Geometry: see drawing. Coordinates: mm, zero at the bounding-box minimum. A direction names the side the tool comes from. Coordinates: 2 decimals unless noted, no trailing zeros. Write each loop counter-clockwise with the first axis right and the second up, starting at its lowest first coordinate (ties: lowest second). Pieces come first, ordered by that corner, then holes. Notation, with made-up numbers: M -29.5,22.25 L -10.5,22.25 A24 ccw -10.5,59.25 Z; hole C 19,19.5 d3. An arc over 180 degrees is marked long. One line per item, written item: value. Start each with the question number.
Item 1: Mould query, pull axis Y, two halves, no side actions, for the marked faces 1, 2 and 3. Classes: released by +Y, released by -Y, zero draft, split by the parting line, or undercut.
Item 2: Cut plane C-C, the plane y = 10. Output: boundary loops of the cut face in (x, z), then the cut area to 3 significant figures.
Item 3: Cut plane D-D, the plane x = 5. Output: boundary loops of the cut face in (y, z), then the cut area to 3 significant figures.
Item 4: Set-up query: the marked faces 4, 5, 6 and 7. Return all of +Z, -Z, +X, -X, +Y, -Y with unobstructed straight access to the full face (end or side cutting, diameter ignored); none if empty.
Item 5: Cut plane A-A, the plane x = 8.75. Output: boundary loops of the cut face in (y, z).
Item 6: Pin query (flat end, axial travel): P1, Ø3.5, axis at y = 9.5, z = 4, coming from the -X side; P2, Ø3, axis at x = 7, y = 6.5, coming from the +Z side; P3, Ø6.5, axis at x = 9.5, y = 9.5, coming from the +Z side; P4, Ø4, axis at x = 15, z = 12.5, coming from the -Y side. Return the tip coordinate at first contact, or that it passes through.
Item 7: Ray query, L1, parallel to X at y = 7.25, z = 18.5; L2, parallel to X at y = 1.5, z = 20.7; L3, parallel to Y at x = 3.25, z = 4. Return the intervals inside material, ascending. Write a range as from..to.
Item 8: Cut plane B-B, the plane z = 21.25. Output: boundary loops of the cut face in (x, y).
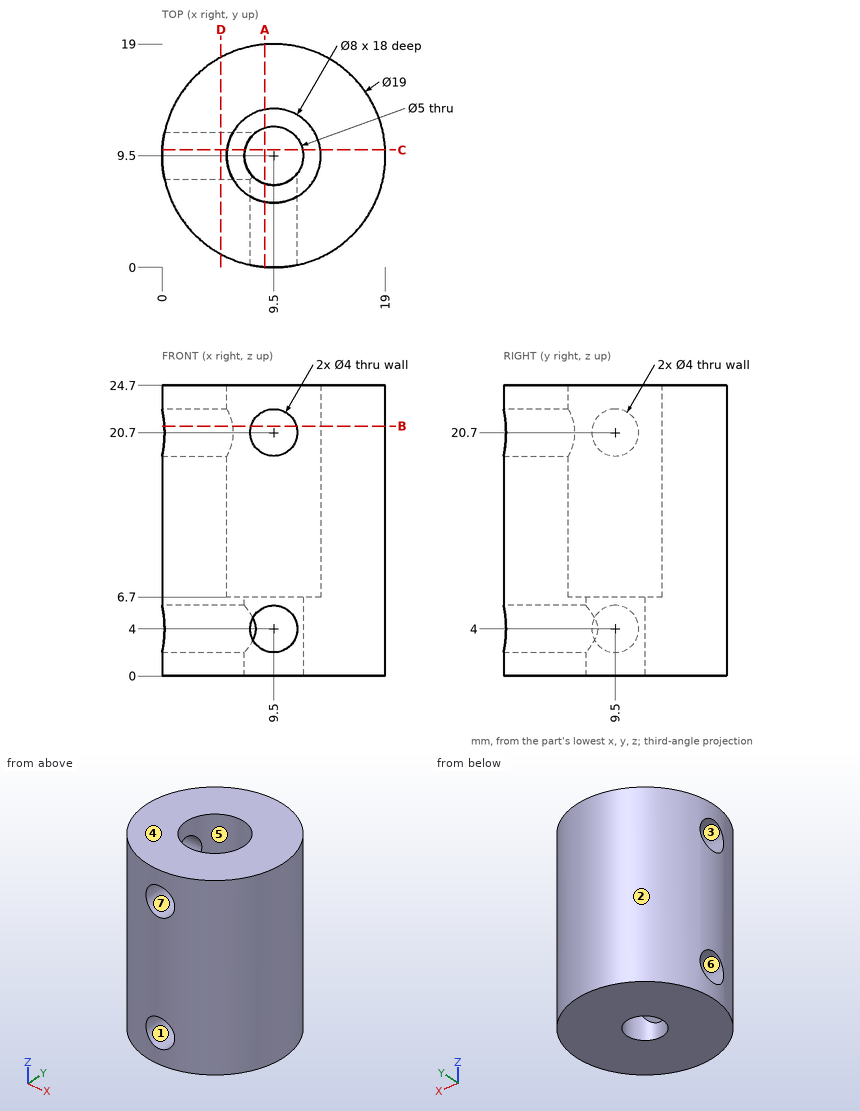
From the geometry:
1. face 1: zero draft
1. face 2: split by the parting line
1. face 3: undercut
2. outline: M 0.01,0 L 7.05,0 L 7.05,2.06 L 0.01,2.06 Z; M 0.01,5.94 L 7.05,5.94 L 7.05,6.7 L 5.53,6.7 L 5.53,18.76 L 0.01,18.76 Z; M 0.01,22.64 L 5.53,22.64 L 5.53,24.7 L 0.01,24.7 Z; M 11.95,0 L 18.99,0 L 18.99,24.7 L 13.47,24.7 L 13.47,6.7 L 11.95,6.7 Z
2. area: 244 mm²
3. outline: M 1.13,0 L 17.87,0 L 17.87,24.7 L 1.13,24.7 Z; hole C 9.5,4 d4; hole C 9.5,20.7 d4
3. area: 388 mm²
4. face 4: +Z, +X, -X, +Y, -Y
4. face 5: +Z
4. face 6: -X
4. face 7: -Y
5. outline: M 0.03,0 L 7.12,0 L 7.12,2.15 L 0.03,2.15 Z; M 0.03,5.85 L 7.12,5.85 L 7.12,6.7 L 5.57,6.7 L 5.57,18.85 L 0.03,18.85 Z; M 0.03,22.55 L 5.57,22.55 L 5.57,24.7 L 0.03,24.7 Z; M 11.88,0 L 18.97,0 L 18.97,24.7 L 13.43,24.7 L 13.43,6.7 L 11.88,6.7 Z
6. P1: stops at x = 11.29
6. P2: stops at z = 24.7
6. P3: stops at z = 6.7
6. P4: stops at y = 0.67
7. L1: x = 0.27..6.19, 12.81..18.73
7. L2: x = 4.38..7.5, 11.5..14.62
7. L3: y = 2.35..7.5, 11.5..16.65
8. outline: M 0.2,7.58 A9.5 ccw 7.58,0.2 L 7.58,5.99 A4 cw 5.99,7.58 Z; M 0.2,11.42 L 5.99,11.42 A4 cw long 11.42,5.99 L 11.42,0.2 A9.5 ccw long Z
